Work out the finished part from the listing and answer in its coordinate system (mm). Coordinates: 2 decimals unless noted, no trailing zeros. Loops run counter-clockwise (first coordinate to the right, second up) from the corner with the lowest first, then second, coordinate; pieces in that order, holes last. Notation, with made-up numbers: (7.5, -37) - (18.5, -37) arc R15 ccw to (18.5, -33) - close; hole circle Ø4 at (30, 81). An arc over 180 degrees is marked (long way). Write each question's results on one line, items separated by ' | '. Start each with the question number.
1. Find the intervals of material crossed by line 1 along X through (y, z) = (1.6, 115); line 2 along X through (y, z) = (0.25, 121), in increasing order. Write a range as [from, to].
2. A cutting plane is placed at C-C on x = -93.5. Determine the outline of the cut face in (y, z) (3 decimals).
3. A cutting plane is placed at A-A on y = 2.5. Determine the outline of the cut face in (x, z).
4. Each of these flat-tipped pins is pushed along its axis until it touches: P1, Ø1, axis at x = -65, y = 1.5, coming from the -Z side; P2, Ø1.6, axis at x = 129, y = 1, coming from the -Z side; P3, Ø1, axis at y = 1, z = 132.5, coming from the -X side; P4, Ø3, axis at x = -115, z = -115, coming from the +Y side (3 decimals). Where does it stop, or does it pass through?
5. A cutting plane is placed at B-B on z = -55.5. Determine the outline of the cut face in (x, y) (3 decimals), then the cut area to 3 significant figures.
from build123d import *

# Parameters (mm, degrees)
SKETCH2_W              = 250
SKETCH2_H              = 250
BASE_DEPTH             = 3.175
SKETCH10_W             = 45
SKETCH10_H             = 3.175
JIGSAW1_DEPTH          = 12.5
SKETCH11_W             = 45
SKETCH11_H             = 3.175
JIGSAW2_DEPTH          = 12.5
SKETCH13_W             = 45
SKETCH13_H             = 3.175
JIGSAW3_DEPTH          = 12.5
SKETCH14_W             = 45
SKETCH14_H             = 3.175
JIGSAW4_DEPTH          = 12.5
STANDOFF_HOLES_D       = 2.5
SKETCH21_R             = 1.25
STANDOFF_HOLES_2_DEPTH = 10


with BuildPart() as part:
    # Sketch2 → Base (new body)
    with BuildSketch(Plane(origin=(0, 0, 0), x_dir=(1, 0, 0), z_dir=(0, 1, 0))):
        Rectangle(SKETCH2_W, SKETCH2_H)
    extrude(amount=BASE_DEPTH)

    # Sketch10 → Jigsaw1 (add)
    with BuildSketch(Plane(origin=(0, 0, -125), x_dir=(-1, 0, 0), z_dir=(0, 0, -1))):
        with Locations((0, 1.5875)):
            Rectangle(SKETCH10_W, SKETCH10_H)
    extrude(amount=JIGSAW1_DEPTH)

    # Sketch11 → Jigsaw2 (add)
    with BuildSketch(Plane.ZY.offset(125)):
        with Locations((0, 1.5875)):
            Rectangle(SKETCH11_W, SKETCH11_H)
    extrude(amount=JIGSAW2_DEPTH)

    # Sketch13 → Jigsaw3 (add)
    with BuildSketch(Plane.XY.offset(125)):
        with Locations((0, 1.5875)):
            Rectangle(SKETCH13_W, SKETCH13_H)
    extrude(amount=JIGSAW3_DEPTH)

    # Sketch14 → Jigsaw4 (add)
    with BuildSketch(Plane(origin=(125, 0, 0), x_dir=(0, 0, -1), z_dir=(1, 0, 0))):
        with Locations((0, 1.5875)):
            Rectangle(SKETCH14_W, SKETCH14_H)
    extrude(amount=JIGSAW4_DEPTH)

    # Standoff Holes (through all)
    with Locations(Plane(origin=(-115, 3.175, -115), x_dir=(0, 0, 1), z_dir=(0, 1, 0))):
        with Locations((0, 0)):
            Hole(STANDOFF_HOLES_D / 2)

    # Sketch21 → Standoff Holes 2 (cut)
    with BuildSketch(Plane(origin=(0, 3.175, 0), x_dir=(1, 0, 0), z_dir=(0, 1, 0))):
        with Locations((115, 115)):
            Circle(SKETCH21_R)
        with Locations((115, -115)):
            Circle(SKETCH21_R)
        with Locations((-115, -115)):
            Circle(SKETCH21_R)
    extrude(amount=-STANDOFF_HOLES_2_DEPTH, mode=Mode.SUBTRACT)


solid = part.part
Values:
1) line 1: [-125, -116.25], [-113.75, 113.75], [116.25, 125] | line 2: [-125, 125]
2) outline: (0, -125) - (3.175, -125) - (3.175, 125) - (0, 125) - close
3) outline: (-137.5, -22.5) - (-125, -22.5) - (-125, -125) - (-22.5, -125) - (-22.5, -137.5) - (22.5, -137.5) - (22.5, -125) - (125, -125) - (125, -22.5) - (137.5, -22.5) - (137.5, 22.5) - (125, 22.5) - (125, 125) - (22.5, 125) - (22.5, 137.5) - (-22.5, 137.5) - (-22.5, 125) - (-125, 125) - (-125, 22.5) - (-137.5, 22.5) - close; hole circle Ø2.5 at (-115, -115); hole circle Ø2.5 at (-115, 115); hole circle Ø2.5 at (115, -115); hole circle Ø2.5 at (115, 115)
4) P1: z = -125 | P2: z = -22.5 | P3: x = -22.5 | P4: y = 3.175
5) outline: (-125, 0) - (125, 0) - (125, 3.175) - (-125, 3.175) - close | area: 794 mm^2
